Geometry check sheet. Reference: the model listing, model coordinates, mm. A direction names the side the tool comes from. Round coordinates to 2 decimals unless told otherwise and drop trailing zeros. Write each loop counter-clockwise with the first axis right and the second up, starting at its lowest first coordinate (ties: lowest second). Pieces come first, ordered by that corner, then holes. Notation, with made-up numbers: (66, 87) -> (93, 87) arc R20 cw to (93, 102) -> close; hole circle Ø7 at (-25.5, 71.5). An arc over 180 degrees is marked (long way). Use a Markdown table: item, result.
```python
from build123d import *

# Parameters (mm, degrees)
F0_W     = 59
F0_H     = 41
F1_DEPTH = 25
F2_R     = 5.5
F2_R_2   = 10
F3_DEPTH = 10
F4_R     = 2
F4_R_2   = 5.5
F5_DEPTH = 10
F6_W     = 10
F6_H     = 23
F7_DEPTH = 10
F8_W     = 5
F8_H     = 25
F9_DEPTH = 10


with BuildPart() as f1:
    # F0 (on Front) → F1 (new body)
    with BuildSketch(Plane.XZ):
        with Locations((2.978919, 0.676766)):
            Rectangle(F0_W, F0_H)
    extrude(amount=F1_DEPTH)

    # F2 (on face) → F3 (join)
    with BuildSketch(Plane.XZ.offset(25)):
        with Locations((-15.521081, 7.676766)):
            Circle(F2_R)
        with Locations((17.478919, 6.176766)):
            Circle(F2_R_2)
    extrude(amount=F3_DEPTH)

    # F4 (on face) → F5 (join)
    with BuildSketch(Plane.XY.offset(21.176766)):
        with Locations((-6.521081, -18)):
            Circle(F4_R)
        with Locations((-15.521081, -12)):
            Circle(F4_R_2)
    extrude(amount=F5_DEPTH)

    # F6 (on face) → F7 (join)
    with BuildSketch(Plane.YZ.offset(32.478919)):
        with Locations((-7, 1.676766)):
            Rectangle(F6_W, F6_H)
    extrude(amount=F7_DEPTH)

    # F8 (on face) → F9 (join)
    with BuildSketch(Plane(origin=(-26.521081, 0, 0), x_dir=(0, -1, 0), z_dir=(-1, 0, 0))):
        with Locations((8.5, 0.676766)):
            Rectangle(F8_W, F8_H)
    extrude(amount=F9_DEPTH)


solid = f1.part
```
(1) Gauge pin test, flat ends, axial feed: pin 1 Ø3 at (x, y) = (35.5, -6.5) entering from -Z; pin 2 Ø1 at (y, z) = (-27.5, 15) entering from +X; pin 3 Ø5.5 at (x, y) = (-32.5, -9) entering from +Z. Record the tip position at first contact, or that the pin passes through.
A:
| item | result |
|---|---|
| pin 1 | stops at z = -9.82 |
| pin 2 | stops at x = 23.02 |
| pin 3 | stops at z = 13.18 |
(2) Access from +Z, -Z, +X, -X, +Y, -Y to the whole of each face (thin tool, end or side, straight path). Record for faces 4 (the face through (22.85, -29.93, 14.61)), 5 (the face through (-6.781, -16.017, 26.107)), 6 (the face through (-31, -11, 1)), 7 (the face through (37, -12, 2)), 8 (the face through (-31, -8, 13.177)).
A:
| item | result |
|---|---|
| face 4 | -Y |
| face 5 | +Z |
| face 6 | +Z, -Z, -X, -Y |
| face 7 | +Z, -Z, +X, -Y |
| face 8 | +Z, -X, +Y, -Y |
(3) Thickness scan on line 1 (Z direction, x = 16, y = -19); line 2 (X direction, y = -17.5, z = -8); line 3 (X direction, y = -7, z = -10.5). Record the ranges inside material, lowest first.
A:
| item | result |
|---|---|
| line 1 | z = -19.82 to 21.18 |
| line 2 | x = -26.52 to 32.48 |
| line 3 | x = -36.52 to 32.48 |
(4) Release check for a two-part mould opening along X. For faces 1 (the face through (37, -7, 13.177)), 2 (the face through (-36.521, -8, 1)), 3 (the face through (-12.56, -29.93, 12.31)) record: +X half, -X half, draft (parallel to the pull), parting line (faces both ways), or undercut.
A:
| item | result |
|---|---|
| face 1 | draft |
| face 2 | -X half |
| face 3 | undercut |
(5) Section check C-C on y = -15. Record the cut outline in (x, z).
A:
| item | result |
|---|---|
| outline | (-26.52, -19.82) -> (32.48, -19.82) -> (32.48, 21.18) -> (-10.91, 21.18) -> (-10.91, 31.18) -> (-20.13, 31.18) -> (-20.13, 21.18) -> (-26.52, 21.18) -> close |
(6) Section check B-B on x = -7.5. Record the cut outline in (y, z).
A:
| item | result |
|---|---|
| outline | (-25, -19.82) -> (0, -19.82) -> (0, 21.18) -> (-16.26, 21.18) -> (-16.26, 31.18) -> (-19.74, 31.18) -> (-19.74, 21.18) -> (-25, 21.18) -> close |
(7) Section check D-D on z = -1. Record the cut outline in (x, y), plus the area to 3 significant figures.
A:
| item | result |
|---|---|
| outline | (-36.52, -11) -> (-26.52, -11) -> (-26.52, -25) -> (10.52, -25) -> (10.52, -35) -> (24.44, -35) -> (24.44, -25) -> (32.48, -25) -> (32.48, -12) -> (42.48, -12) -> (42.48, -2) -> (32.48, -2) -> (32.48, 0) -> (-26.52, 0) -> (-26.52, -6) -> (-36.52, -6) -> close |
| area | 1,760 mm2 |
(8) Section check A-A on z = 23. Record the cut outline in (x, y), plus the area to 3 significant figures.
A:
| item | result |
|---|---|
| outline | circle Ø11 at (-15.52, -12); circle Ø4 at (-6.52, -18) |
| area | 108 mm2 |
